```python
from build123d import *

# Parameters (mm, degrees)
F0_R        = 25
F0_R_2      = 20
F0_R_3      = 17.5
F1_DEPTH    = 25.4
F2_DEPTH    = 55.4
F4_DEPTH    = 30
F5_T2_ANGLE = 128.886649626
F5_T4_ANGLE = 129.1121145727
F5_T6_ANGLE = 128.886649626
F5_T8_ANGLE = 129.1121145727
F6_R        = 4


# Not quite as in the source:
# - a fillet or chamfer that OpenCascade refuses, or shapes differently, is made with other operations: its cross-section is extruded or revolved along the edge and cut away or added


with BuildPart() as f1:
    # F0 (on Top) → F1 (new body)
    with BuildSketch(Plane.XY):
        Circle(F0_R)
        Circle(F0_R_2, mode=Mode.SUBTRACT)
        Circle(F0_R_2)
        Circle(F0_R_3, mode=Mode.SUBTRACT)
    extrude(amount=F1_DEPTH)

    # F0 (on Top) → F2 (join)
    with BuildSketch(Plane.XY):
        Circle(F0_R_2)
        Circle(F0_R_3, mode=Mode.SUBTRACT)
    extrude(amount=F2_DEPTH)

    # F3 (on face) → F4 (cut)
    with BuildSketch(Plane.XY.offset(55.4)):
        with BuildLine():
            Line((0, 20), (0, 17.5))
            ThreePointArc((0, 17.5), (0.5, 17.4928556845), (0.9995917534, 17.4714285714))
            Line((0.9995917534, 17.4714285714), (1.1423905753, 19.9673469388))
            ThreePointArc((1.1423905753, 19.9673469388), (0.5714285714, 19.991835068), (0, 20))
        make_face()
        with BuildLine():
            Line((20, 0), (17.5, 0))
            ThreePointArc((17.5, 0), (17.4928556845, -0.5), (17.4714285714, -0.9995917534))
            Line((17.4714285714, -0.9995917534), (19.9626986738, -1.2209265568))
            ThreePointArc((19.9626986738, -1.2209265568), (19.9906724934, -0.6107481163), (20, 0))
        make_face()
        with BuildLine():
            ThreePointArc((-17.5, 0), (-17.4928556845, 0.5), (-17.4714285714, 0.9995917534))
            Line((-17.4714285714, 0.9995917534), (-19.9626986738, 1.2209265568))
            ThreePointArc((-19.9626986738, 1.2209265568), (-19.9906724934, 0.6107481163), (-20, 0))
            Line((-20, 0), (-17.5, 0))
        make_face()
        with BuildLine():
            ThreePointArc((0, -17.5), (-0.5, -17.4928556845), (-0.9995917534, -17.4714285714))
            Line((-0.9995917534, -17.4714285714), (-1.1423905753, -19.9673469388))
            ThreePointArc((-1.1423905753, -19.9673469388), (-0.5714285714, -19.991835068), (0, -20))
            Line((0, -20), (0, -17.5))
        make_face()
    extrude(amount=-F4_DEPTH, mode=Mode.SUBTRACT)

    # F5: fillet of radius 3 on 4 edges, made by hand

    # F5_s1 → F5_t2 (revolve, cut)
    with BuildSketch(Plane(origin=(0, 0, 0), x_dir=(0, 0, 1), z_dir=(0.9323663261, -0.3615149152, 0))):
        with BuildLine():
            ThreePointArc((52.4419601084, -20), (54.3784517816, -19.2912878475), (55.4, -17.5))
            Line((55.4, -17.5), (55.4, -20))
            Line((55.4, -20), (52.4419601084, -20))
        make_face()
    revolve(axis=Axis((0, 0, 55.4), (0, 0, 1)), revolution_arc=F5_T2_ANGLE, mode=Mode.SUBTRACT)

    # F5_s3 → F5_t4 (revolve, cut)
    with BuildSketch(Plane(origin=(0, 0, 0), x_dir=(0, 0, 1), z_dir=(0.3615155829, 0.9323660672, 0))):
        with BuildLine():
            ThreePointArc((52.4419601084, -20), (54.3784517816, -19.2912878475), (55.4, -17.5))
            Line((55.4, -17.5), (55.4, -20))
            Line((55.4, -20), (52.4419601084, -20))
        make_face()
    revolve(axis=Axis((0, 0, 55.4), (0, 0, 1)), revolution_arc=F5_T4_ANGLE, mode=Mode.SUBTRACT)

    # F5_s5 → F5_t6 (revolve, cut)
    with BuildSketch(Plane(origin=(0, 0, 0), x_dir=(0, 0, 1), z_dir=(-0.9323663261, 0.3615149152, 0))):
        with BuildLine():
            ThreePointArc((52.4419601084, -20), (54.3784517816, -19.2912878475), (55.4, -17.5))
            Line((55.4, -17.5), (55.4, -20))
            Line((55.4, -20), (52.4419601084, -20))
        make_face()
    revolve(axis=Axis((0, 0, 55.4), (0, 0, 1)), revolution_arc=F5_T6_ANGLE, mode=Mode.SUBTRACT)

    # F5_s7 → F5_t8 (revolve, cut)
    with BuildSketch(Plane(origin=(0, 0, 0), x_dir=(0, 0, 1), z_dir=(-0.3615155829, -0.9323660672, 0))):
        with BuildLine():
            ThreePointArc((52.4419601084, -20), (54.3784517816, -19.2912878475), (55.4, -17.5))
            Line((55.4, -17.5), (55.4, -20))
            Line((55.4, -20), (52.4419601084, -20))
        make_face()
    revolve(axis=Axis((0, 0, 55.4), (0, 0, 1)), revolution_arc=F5_T8_ANGLE, mode=Mode.SUBTRACT)

    # F6
    f6_edges = [f1.edges().sort_by_distance(p)[0] for p in [
        (-25, 0, 0),
    ]]
    fillet(f6_edges, radius=F6_R)


solid = f1.part
```
CAD build for the part. Positions are in the model's coordinates, mm. A direction names the side the tool comes from. Round coordinates to 2 decimals unless told otherwise and drop trailing zeros. Loops run counter-clockwise (first coordinate to the right, second up) from the corner with the lowest first, then second, coordinate; pieces in that order, holes last. Notation, with made-up numbers: M 9.25,-3.5 L 21.25,-3.5 A24 ccw 21.25,23.5 Z; hole C 22,77.5 d9. An arc over 180 degrees is marked long. Use a Markdown table: item, result. Add a question column.
(1) Cut at A-A (z = 50). Give the cut face in (x, y).
(2) Flat gauge pins, fed straight in: pin 1 (8 mm diameter, centred on x = 18, z = 21, fed in from -Y); pin 2 (3 mm diameter, centred on y = 4.5, z = 11.5, fed in from +X); pin 3 (2 mm diameter, centred on x = -18.5, z = 34, fed in from +Y); pin 4 (2 mm diameter, centred on x = -13, y = 11, fed in from +Z). Where does each tip first touch, or does it go through?
(3) Pull direction X, two halves, no side cores. Call faces 1 (the face through (0, 19, 41)), 2 (the face through (1.07, 18.7, 40.61)), 3 (the face through (13.55, -14.71, 38.73)), 4 (the face through (-13.55, 14.71, 38.73)): +X half, -X half, draft (parallel to the pull), parting line (faces both ways), or undercut.
(4) Which spindle directions (+Z, -Z, +X, -X, +Y, -Y) get a long thin tool onto all of the face, cutting with end or side? Do faces 5 (the face through (-14.685, -13.577, 38.732)), 6 (the face through (-19, -7, 25.4)), 7 (the face through (-18.7, 1.11, 40.61)), 8 (the face through (0, -19, 41)). Say none if no direction does.
(5) Drill centre lines: line 1 (Y direction, x = -5, z = 30.5); line 2 (Y direction, x = 0, z = 19); line 3 (X direction, y = 3, z = 33.5). Where is each one in solid material? Low to high.
(6) Cut at B-B (z = 22.5). Give the cut face in (x, y), and give its area (3 significant figures).
Geometry says:
| question | item | result |
|---|---|---|
| 1 | outline | M -20,0 A20 ccw -1.14,-19.97 L -1,-17.47 A17.5 cw -17.5,0 Z; M -19.96,1.22 L -17.47,1 A17.5 cw 0,17.5 L 0,20 A20 ccw Z; M 0,-20 A20 ccw 19.96,-1.22 L 17.47,-1 A17.5 cw 0,-17.5 Z; M 1,17.47 A17.5 cw 17.5,0 L 20,0 A20 ccw 1.14,19.97 Z |
| 2 | pin 1 | stops at y = -20.71 |
| 2 | pin 2 | stops at x = 24.82 |
| 2 | pin 3 | stops at y = 9.68 |
| 2 | pin 4 | stops at z = 55.4 |
| 3 | face 1 | undercut |
| 3 | face 2 | undercut |
| 3 | face 3 | +X half |
| 3 | face 4 | -X half |
| 4 | face 5 | +Z, -X, -Y |
| 4 | face 6 | +Z |
| 4 | face 7 | +Z, -X |
| 4 | face 8 | +Z, -Y |
| 5 | line 1 | y = -19.36 to -16.77, 16.77 to 19.36 |
| 5 | line 2 | y = -25 to -17.5, 17.5 to 25 |
| 5 | line 3 | x = -19.77 to -17.24, 17.24 to 19.77 |
| 6 | outline | C 0,0 d50; hole C 0,0 d35 |
| 6 | area | 1,000 mm² |
